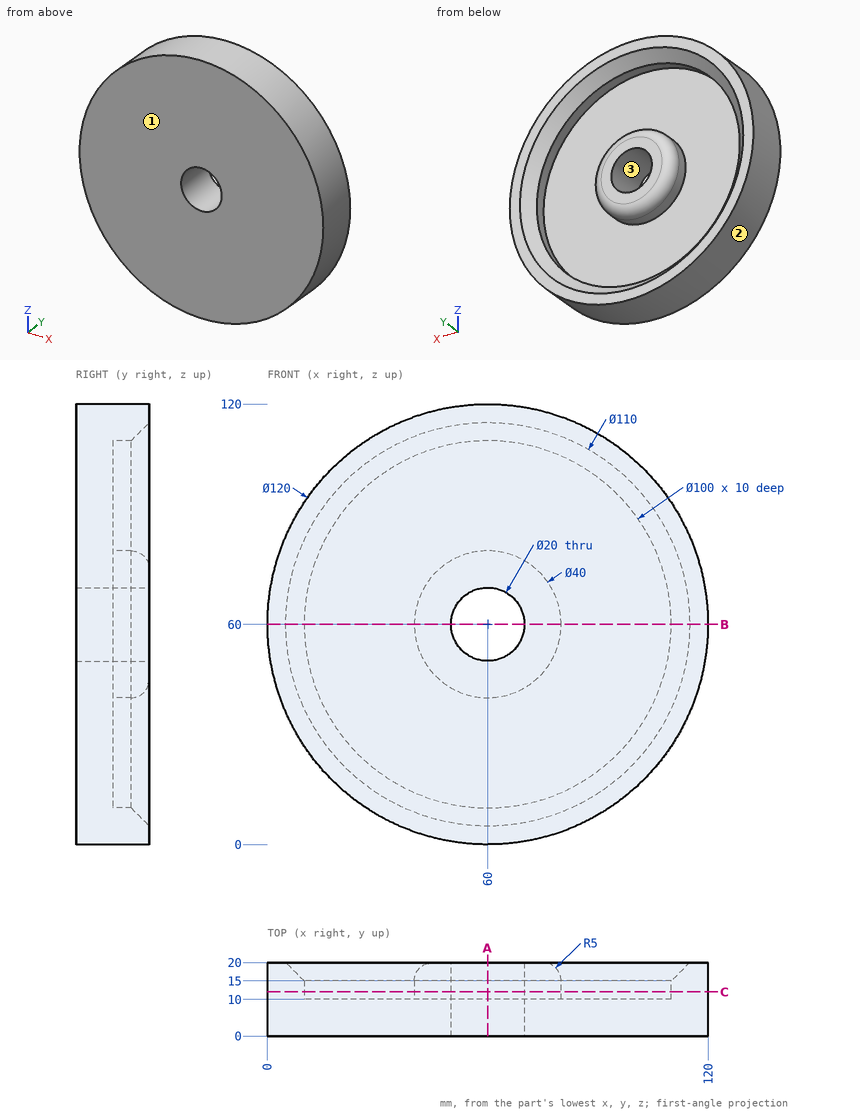
Geometry check sheet. Reference: drawing and pictorial views, mm from the part's lowest x, y, z. Give positions to 0.01 mm unless a question says otherwise; leave off trailing zeros. Write each loop counter-clockwise with the first axis right and the second up, starting at its lowest first coordinate (ties: lowest second). Pieces come first, ordered by that corner, then holes. Notation, with made-up numbers: (50.25, 47.5) - (70.25, 47.5) arc R20 cw to (70.25, 77.5) - close; hole circle Ø9 at (48.5, 9). An arc over 180 degrees is marked (long way). Use a Markdown table: item, result.
Q1. Section check A-A, the plane x = 60. Enter the section's corners in (y, z), then the cut area to 3 significant figures.
Computed:
| item | result |
|---|---|
| outline | (0, 0) - (20, 0) - (20, 5) - (15, 10) - (10, 10) - (10, 40) - (15, 40) arc R5 ccw to (20, 45) - (20, 50) - (0, 50) - close; (0, 70) - (20, 70) - (20, 75) arc R5 ccw to (15, 80) - (10, 80) - (10, 110) - (15, 110) - (20, 115) - (20, 120) - (0, 120) - close |
| area | 1,360 mm² |
Q2. Thickness scan on L1, parallel to Z at x = 60, y = 11.25; L2, parallel to Z at x = 60, y = 5.75; L3, parallel to X at y = 11.5, z = 56. Record the ranges inside material, lowest first. Write a range as [from, to].
Computed:
| item | result |
|---|---|
| L1 | z = [0, 10], [40, 50], [70, 80], [110, 120] |
| L2 | z = [0, 50], [70, 120] |
| L3 | x = [0.13, 10.16], [40.4, 50.83], [69.17, 79.6], [109.84, 119.87] |
Q3. Go/stop test with flat-tipped pins: P1, Ø2, axis at y = 11.5, z = 41.5, coming from the +X side; P2, Ø1, axis at x = 87.5, y = 5.5, coming from the +Z side; P3, Ø8, axis at x = 21, z = 87, coming from the +Y side. Record where each tip stops, or that it passes through.
Computed:
| item | result |
|---|---|
| P1 | stops at x = 117.39 |
| P2 | stops at z = 113.58 |
| P3 | stops at y = 16.43 |
Q4. Section check C-C, the plane y = 12. Enter the section's corners in (x, z).
Computed:
| item | result |
|---|---|
| outline | circle Ø120 at (60, 60); circle Ø40 at (60, 60); hole circle Ø100 at (60, 60); hole circle Ø20 at (60, 60) |
Q5. Draft check along Z on the marked faces 1, 2 and 3. Enter one of: pulls with the +Z half, pulls with the -Z half, needs draft (parallel to the pull), parting line crosses it, or undercut.
Computed:
| item | result |
|---|---|
| face 1 | needs draft |
| face 2 | parting line crosses it |
| face 3 | undercut |
Q6. Section check B-B, the plane z = 60. Enter the section's corners in (x, y), then the cut area to 3 significant figures.
Computed:
| item | result |
|---|---|
| outline | (0, 0) - (50, 0) - (50, 20) - (45, 20) arc R5 ccw to (40, 15) - (40, 10) - (10, 10) - (10, 15) - (5, 20) - (0, 20) - close; (70, 0) - (120, 0) - (120, 20) - (115, 20) - (110, 15) - (110, 10) - (80, 10) - (80, 15) arc R5 ccw to (75, 20) - (70, 20) - close |
| area | 1,360 mm² |
